Check sheet for the modelled part. Datum: model origin and axes. Units: mm. A direction names the side the tool comes from. Round coordinates to 2 decimals unless told otherwise and drop trailing zeros. Order: outer loops, then holes, each group sorted by start corner. A loop starts at its lowest first (then second) coordinate and runs counter-clockwise, first axis right, second up.
from build123d import *

# Parameters (mm, degrees)
SKETCH1_W           = 211
SKETCH1_H           = 121
BOSS_EXTRUDE1_DEPTH = 12
SKETCH2_W           = 201
SKETCH2_H           = 111
CUT_EXTRUDE1_DEPTH  = 7
SKETCH3_R           = 32
CUT_EXTRUDE2_DEPTH  = 244.52823245
BOSS_EXTRUDE2_DEPTH = 50
SKETCH5_R           = 1.6
CUT_EXTRUDE3_DEPTH  = 6
FILLET1_R           = 4
FILLET2_R           = 10


with BuildPart() as part:
    # Sketch1 → Boss-Extrude1 (new body)
    with BuildSketch(Plane(origin=(0, 0, 0), x_dir=(1, 0, 0), z_dir=(0, 1, 0))):
        with Locations((105.5, 60.5)):
            Rectangle(SKETCH1_W, SKETCH1_H)
    extrude(amount=BOSS_EXTRUDE1_DEPTH)

    # Sketch2 → Cut-Extrude1 (cut)
    with BuildSketch(Plane.XZ):
        with Locations((105.5, -60.5)):
            Rectangle(SKETCH2_W, SKETCH2_H)
    extrude(amount=-CUT_EXTRUDE1_DEPTH, mode=Mode.SUBTRACT)

    # Sketch3 → Cut-Extrude2 (cut, through all)
    with BuildSketch(Plane(origin=(0, 12, 0), x_dir=(1, 0, 0), z_dir=(0, 1, 0))):
        with Locations(Location((105.5, 60.5, 0), (0, 0, 270))):
            Circle(SKETCH3_R)
    extrude(amount=-CUT_EXTRUDE2_DEPTH, mode=Mode.SUBTRACT)

    # Sketch4 → Boss-Extrude2 (add)
    with BuildSketch(Plane(origin=(0, 12, 0), x_dir=(1, 0, 0), z_dir=(0, 1, 0))):
        with BuildLine():
            ThreePointArc((140.957721303, 45.5), (67, 60.5), (140.957721303, 75.5))
            Line((140.957721303, 75.5), (145.775366264, 75.5))
            Line((145.775366264, 75.5), (146.331972766, 75.5))
            ThreePointArc((146.331972766, 75.5), (145.74451839, 77.011472968), (145.101136347, 78.5))
            ThreePointArc((145.101136347, 78.5), (62, 60.5), (145.101136347, 42.5))
            ThreePointArc((145.101136347, 42.5), (145.74451839, 43.988527032), (146.331972766, 45.5))
            Line((146.331972766, 45.5), (145.775366264, 45.5))
            Line((145.775366264, 45.5), (140.957721303, 45.5))
        make_face()
        with BuildLine():
            Line((146.331972766, 75.5), (145.775366264, 75.5))
            Line((145.775366264, 75.5), (145.775366264, 45.5))
            Line((145.775366264, 45.5), (146.331972766, 45.5))
            ThreePointArc((146.331972766, 45.5), (147.885391427, 50.715900981), (148.775366264, 56.084949069))
            Line((148.775366264, 56.084949069), (148.775366264, 64.915050931))
            ThreePointArc((148.775366264, 64.915050931), (147.885391427, 70.284099019), (146.331972766, 75.5))
        make_face()
        with BuildLine():
            ThreePointArc((145.101136347, 78.5), (145.74451839, 77.011472968), (146.331972766, 75.5))
            Line((146.331972766, 75.5), (148.775366264, 75.5))
            Line((148.775366264, 75.5), (148.775366264, 78.5))
            Line((148.775366264, 78.5), (145.101136347, 78.5))
        make_face()
        with BuildLine():
            Line((148.775366264, 75.5), (146.331972766, 75.5))
            ThreePointArc((146.331972766, 75.5), (147.885391427, 70.284099019), (148.775366264, 64.915050931))
            Line((148.775366264, 64.915050931), (148.775366264, 75.5))
        make_face()
        with BuildLine():
            ThreePointArc((148.775366264, 56.084949069), (147.885391427, 50.715900981), (146.331972766, 45.5))
            Line((146.331972766, 45.5), (148.775366264, 45.5))
            Line((148.775366264, 45.5), (148.775366264, 56.084949069))
        make_face()
        with BuildLine():
            Line((148.775366264, 45.5), (146.331972766, 45.5))
            ThreePointArc((146.331972766, 45.5), (145.74451839, 43.988527032), (145.101136347, 42.5))
            Line((145.101136347, 42.5), (148.775366264, 42.5))
            Line((148.775366264, 42.5), (148.775366264, 45.5))
        make_face()
    extrude(amount=BOSS_EXTRUDE2_DEPTH)

    # Sketch5 → Cut-Extrude3 (cut)
    with BuildSketch(Plane(origin=(148.775366264, 0, 0), x_dir=(0, 0, -1), z_dir=(1, 0, 0))):
        with Locations((52.5, 52)):
            Circle(SKETCH5_R)
        with Locations((68.5, 52)):
            Circle(SKETCH5_R)
        with Locations((68.5, 17)):
            Circle(SKETCH5_R)
        with Locations((52.5, 17)):
            Circle(SKETCH5_R)
    extrude(amount=-CUT_EXTRUDE3_DEPTH, mode=Mode.SUBTRACT)

    # Fillet1
    fillet1_edges = [part.edges().sort_by_distance(p)[0] for p in [
        (146.938251306, 12, -42.5),
        (145.101136347, 37, -42.5),
        (62, 12, -60.5),
        (145.101136347, 37, -78.5),
        (146.938251306, 12, -78.5),
    ]]
    fillet(fillet1_edges, radius=FILLET1_R)

    # Fillet2
    fillet2_edges = [part.edges().sort_by_distance(p)[0] for p in [
        (5, 3.5, -116),
        (5, 3.5, -5),
        (206, 3.5, -5),
        (206, 3.5, -116),
        (0, 6, -121),
        (211, 6, -121),
        (211, 6, 0),
        (0, 6, 0),
    ]]
    fillet(fillet2_edges, radius=FILLET2_R)


solid = part.part
1) Gauge pin test, flat ends, axial feed: pin 1 (1.3 mm diameter, centred on x = 148.5, y = 35.5, fed in from +Z); pin 2 (1.5 mm diameter, centred on x = 155.5, z = -27, fed in from -Y); pin 3 (1 mm diameter, centred on y = 14, z = -78.5, fed in from -X). Record the tip position at first contact, or that the pin passes through.
2) Sectioned sample at A-A on x = 156.5. Record the cut outline in (y, z), and give its area (3 significant figures).
3) Scan lines: line 1 (Y direction, x = 146.5, z = -68.5); line 2 (X direction, y = 3, z = -86); line 3 (X direction, y = 11, z = -60). Record each from-to range of solid material in increasing order.
4) Set-up check for faces 4 (the face through (89, 62, -25)), 5 (the face through (112, 12, -92)), 6 (the face through (104, 3, -116)): record each of +Z, -Z, +X, -X, +Y, -Y from which the full face is reachable in a straight line by a thin tool's end or side.
5) Draft check along X on faces 1 (the face through (8.01, 3.55, -7.85)), 2 (the face through (0, 6, -60)), 3 (the face through (207.99, 6.08, -118.15)). Enter one of: pulls with the +X half, pulls with the -X half, needs draft (parallel to the pull), parting line crosses it, or undercut.
Values found:
1. pin 1: stops at z = -42.5
1. pin 2: stops at y = 7
1. pin 3: stops at x = 64.88
2. outline: (0, -121) - (12, -121) - (12, 0) - (0, 0) - (0, -5) - (7, -5) - (7, -116) - (0, -116) - close
2. area: 675 mm2
3. line 1: y = 7 to 15.4, 18.6 to 50.4, 53.6 to 62
3. line 2: x = 0 to 5, 206 to 211
3. line 3: x = 0 to 73.5, 137.5 to 211
4. face 4: +Z, -Z, +X, -X, +Y
4. face 5: +Y
4. face 6: -Y
5. face 1: undercut
5. face 2: pulls with the -X half
5. face 3: pulls with the +X half
